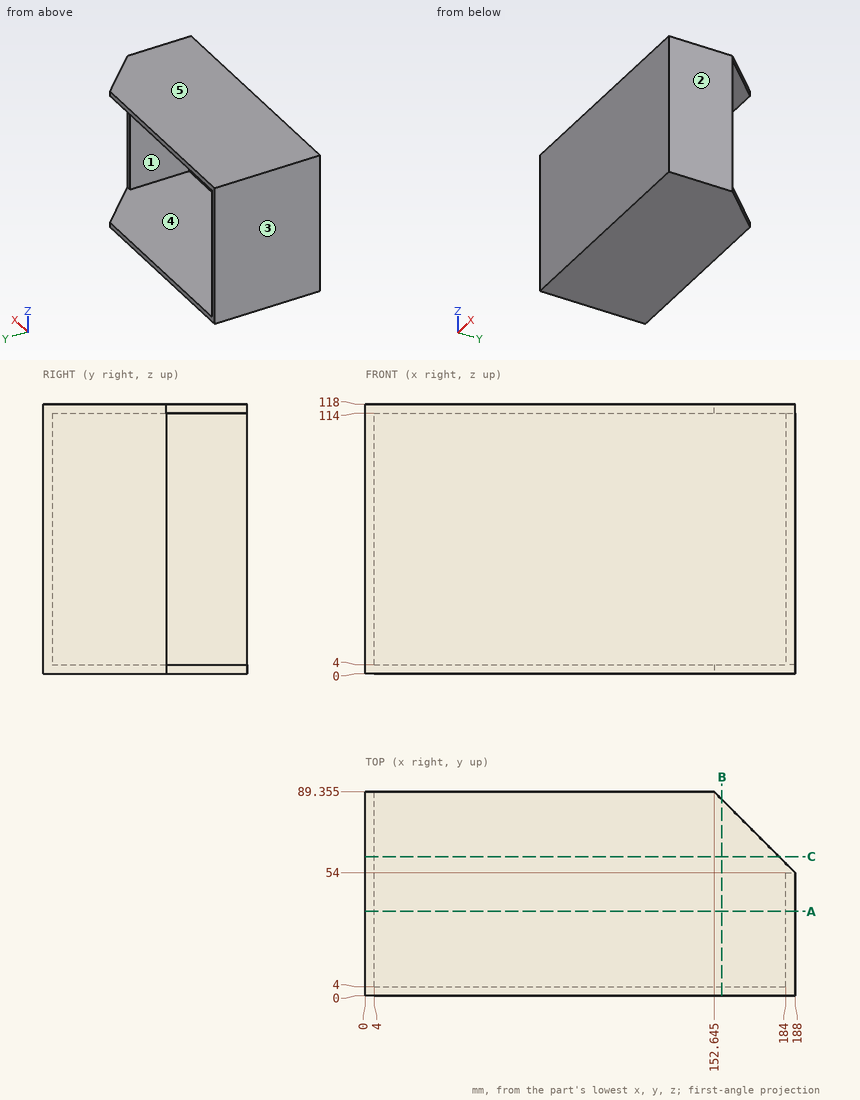
Here's the drawing with two shaded views (mm, measured from the low corner). I have some questions. A direction names the side the tool comes from. Coordinates: 2 decimals unless noted, no trailing zeros. Write each loop counter-clockwise with the first axis right and the second up, starting at its lowest first coordinate (ties: lowest second). Pieces come first, ordered by that corner, then holes.
Item 1: If we mould it in two halves opening along X, with no side actions, what happens to the marked faces 3, 4 and 5? For each: +X half, -X half, draft (parallel to the pull), parting line (faces both ways), or undercut.
Item 2: On a 3-axis mill with a long thin cutter (end or side, diameter ignored), from which of +Z, -Z, +X, -X, +Y, -Y can I reach the whole of each face in a straight line? I mean the marked faces 1 and 2. Say none if no direction works.
Item 3: If I drill on line 1 (Z direction, x = 46, y = 30.5); line 2 (X direction, y = 26, z = 104.5); line 3 (Y direction, x = 35.5, z = 41), over which ranges is the centre line in solid material (lowest first)?
Item 4: I want a section at A-A on y = 37. Write out the boundary of the cut face in (x, z).
Item 5: I want a section at B-B on x = 156. Write out the boundary of the cut face in (y, z), and give its area (3 significant figures).
Item 6: Will this pin go through, and if not, where does the flat tip stop? pin 1 (1.2 mm diameter, centred on x = 186, z = 48.5, fed in from +Y).
Item 7: I want a section at C-C on y = 61. Write out the boundary of the cut face in (x, z), and give its area (3 significant figures).
Findings below:
1. face 3: -X half
1. face 4: undercut
1. face 5: draft
2. face 1: +Y
2. face 2: +Z, -Z, +X, +Y, -Y
3. line 1: z = 0 to 4, 114 to 118
3. line 2: x = 0 to 4, 184 to 188
3. line 3: y = 0 to 4
4. outline: (0, 0) - (188, 0) - (188, 118) - (0, 118) - close; hole (4, 4) - (184, 4) - (184, 114) - (4, 114) - close
5. outline: (0, 0) - (86, 0) - (86, 4) - (4, 4) - (4, 114) - (86, 114) - (86, 118) - (0, 118) - close
5. area: 1,130 mm2
6. pin 1: stops at y = 54
7. outline: (0, 0) - (181, 0) - (181, 4) - (4, 4) - (4, 114) - (181, 114) - (181, 118) - (0, 118) - close
7. area: 1,890 mm2
